The drawing under review shows one solid part. Ordinate dimensions are in mm from its lowest x, y, z. A direction names the side the tool comes from. Give positions to 0.01 mm unless a question says otherwise; leave off trailing zeros. Write each loop counter-clockwise with the first axis right and the second up, starting at its lowest first coordinate (ties: lowest second). Pieces come first, ordered by that corner, then holes.
Q1. For line 1 (Y direction, x = 32.5, z = 2.3); line 2 (X direction, y = 7, z = 2); line 3 (Z direction, x = 36.5, y = 21.5), list the stretches that pass through material, from the lowest coordinate up.
Q2. We need section C-C (x = 20). Write out the cut boundary in (y, z).
Q3. We need section A-A (y = 20). Write out the cut boundary in (x, z).
Q4. Insertion check: P1, Ø2, axis at y = 13, z = 12.5, coming from the -X side; P2, Ø1, axis at y = 8.5, z = 12, coming from the +X side; P3, Ø1, axis at x = 16.5, z = 10, coming from the -Y side. Each pin has a flat end and moves straight along its axis. Give the tip position at first contact, or say it passes through.
Q5. We need section B-B (z = 19). Write out the cut boundary in (x, y), then the cut area to 3 significant figures.
Q6. Machinability: for the marked faces 1 and 2, which of the approach directions +Z, -Z, +X, -X, +Y, -Y give a long, thin tool a straight path to every point of the face, cutting with its end or side? Answer none if there is none.
Q7. Mouldability with a two-part tool opening along Y and no side actions: class the marked faces 3, 4 and 5 as released by +Y, released by -Y, zero draft, split by the parting line, or undercut.
Q8. We need section D-D (x = 8.5). Give the number of separate pieces and of enclosed holes in the cut face, then the cut area to 3 significant figures.
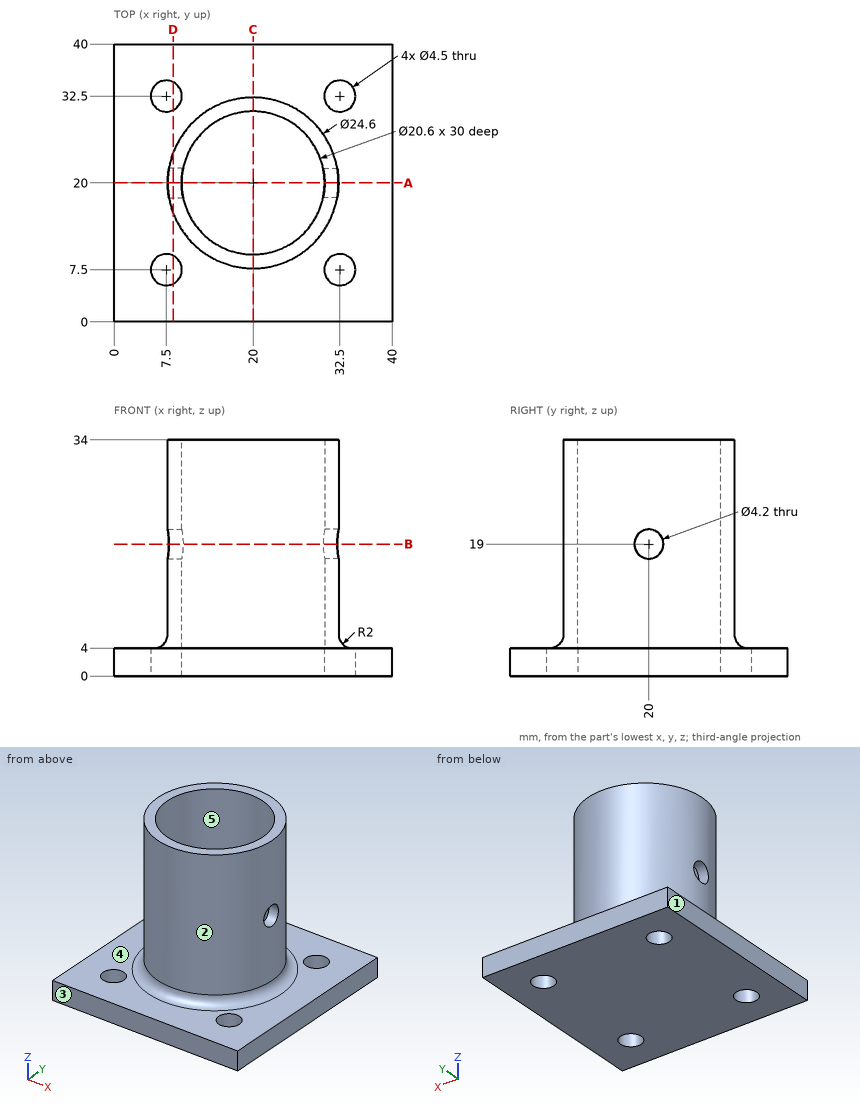
Computed:
1. line 1: y = 0 to 5.25, 9.75 to 30.25, 34.75 to 40
1. line 2: x = 0 to 5.31, 9.69 to 30.31, 34.69 to 40
1. line 3: z = 0 to 4
2. outline: (0, 0) - (40, 0) - (40, 4) - (34.3, 4) arc R2 cw to (32.3, 6) - (32.3, 34) - (30.3, 34) - (30.3, 4) - (9.7, 4) - (9.7, 34) - (7.7, 34) - (7.7, 6) arc R2 cw to (5.7, 4) - (0, 4) - close
3. outline: (0, 0) - (40, 0) - (40, 4) - (34.3, 4) arc R2 cw to (32.3, 6) - (32.3, 16.9) - (30.3, 16.9) - (30.3, 4) - (9.7, 4) - (9.7, 16.9) - (7.7, 16.9) - (7.7, 6) arc R2 cw to (5.7, 4) - (0, 4) - close; (7.7, 21.1) - (9.7, 21.1) - (9.7, 34) - (7.7, 34) - close; (30.3, 21.1) - (32.3, 21.1) - (32.3, 34) - (30.3, 34) - close
4. P1: stops at x = 9.26
4. P2: stops at x = 25.5
4. P3: stops at y = 8.07
5. outline: (7.88, 17.9) arc R12.3 ccw to (32.12, 17.9) - (30.08, 17.9) arc R10.3 cw to (9.92, 17.9) - close; (7.88, 22.1) - (9.92, 22.1) arc R10.3 cw to (30.08, 22.1) - (32.12, 22.1) arc R12.3 ccw to start
5. area: 125 mm2
6. face 1: +Z, -Z, -X, +Y, -Y
6. face 2: +Z
7. face 3: released by -Y
7. face 4: zero draft
7. face 5: undercut
8. separate pieces: 3
8. enclosed holes: 1
8. area: 380 mm2
